Geometry check sheet. Reference: the model listing, model coordinates, mm. A direction names the side the tool comes from. Round coordinates to 2 decimals unless told otherwise and drop trailing zeros. Write each loop counter-clockwise with the first axis right and the second up, starting at its lowest first coordinate (ties: lowest second). Pieces come first, ordered by that corner, then holes. Notation, with made-up numbers: M 42.25,-24.5 L 48.25,-24.5 A31 cw 48.25,5.5 Z; hole C 9,66.5 d4. An arc over 180 degrees is marked long. Use a Markdown table: item, result.
```python
from build123d import *

# Parameters (mm, degrees)
BOSS_EXTRUDE1_DEPTH = 80
SKETCH2_R           = 25
CUT_EXTRUDE1_DEPTH  = 161
SKETCH3_R           = 15
CUT_EXTRUDE2_DEPTH  = 10


with BuildPart() as part:
    # Sketch1 → Boss-Extrude1 (new body)
    with BuildSketch(Plane.XY):
        Polygon((0, 0), (0, 480), (800, 480), (800, 400), (80, 400), (80, 0), align=None)
    extrude(amount=BOSS_EXTRUDE1_DEPTH)

    # Sketch2 → Cut-Extrude1 (cut)
    with BuildSketch(Plane.XY.offset(80)):
        with Locations((750, 440)):
            Circle(SKETCH2_R)
    extrude(amount=-CUT_EXTRUDE1_DEPTH, mode=Mode.SUBTRACT)

    # Sketch3 → Cut-Extrude2 (cut)
    with BuildSketch(Plane.XZ):
        with Locations(Location((40, 40, 0), (0, 0, 270))):
            Circle(SKETCH3_R)
    extrude(amount=-CUT_EXTRUDE2_DEPTH, mode=Mode.SUBTRACT)


solid = part.part
```
Item 1: Go/stop test with flat-tipped pins: pin 1 (8 mm diameter, centred on x = 398.5, z = 68, fed in from -Y); pin 2 (24 mm diameter, centred on y = 136, z = 44, fed in from +X); pin 3 (24 mm diameter, centred on x = 40, z = 40, fed in from -Y). Record where each tip stops, or that it passes through.
Outcome:
| item | result |
|---|---|
| pin 1 | stops at y = 400 |
| pin 2 | stops at x = 80 |
| pin 3 | stops at y = 10 |
Item 2: Cross-section at B-B, the plane z = 40. Record the cut outline in (x, y).
Outcome:
| item | result |
|---|---|
| outline | M 0,0 L 25,0 L 25,10 L 55,10 L 55,0 L 80,0 L 80,400 L 800,400 L 800,480 L 0,480 Z; hole C 750,440 d50 |
Item 3: Mould release check, pull along X, two halves, no side actions. Record for faces 4 (the face through (763.44, 461.08, 40.56)), 5 (the face through (800, 441, 39)), 6 (the face through (283, 401, 0)), 7 (the face through (0, 237, 39)): +X half, -X half, draft (parallel to the pull), parting line (faces both ways), or undercut.
Outcome:
| item | result |
|---|---|
| face 4 | undercut |
| face 5 | +X half |
| face 6 | draft |
| face 7 | -X half |
Item 4: Access from +Z, -Z, +X, -X, +Y, -Y to the whole of each face (thin tool, end or side, straight path). Record for faces 1 (the face through (50.138, 4.93, 51.056)), 2 (the face through (80, 203, 39)), 3 (the face through (394, 480, 39)).
Outcome:
| item | result |
|---|---|
| face 1 | -Y |
| face 2 | +Z, -Z, +X, -Y |
| face 3 | +Z, -Z, +X, -X, +Y |
Item 5: Material ranges on line 1 along X through (y, z) = (7.25, 40); line 2 along Y through (x, z) = (750, 47); line 3 along Y through (x, z) = (507, 53.5), recorded low to high. Write a range as from..to.
Outcome:
| item | result |
|---|---|
| line 1 | x = 0..25, 55..80 |
| line 2 | y = 400..415, 465..480 |
| line 3 | y = 400..480 |
Item 6: Cross-section at A-A, the plane y = 425. Record the cut outline in (x, z), and give its area (3 significant figures).
Outcome:
| item | result |
|---|---|
| outline | M 0,0 L 730,0 L 730,80 L 0,80 Z; M 770,0 L 800,0 L 800,80 L 770,80 Z |
| area | 60,800 mm2 |
Item 7: Cross-section at D-D, the plane y = 126. Record the cut outline in (x, z), and give its area (3 significant figures).
Outcome:
| item | result |
|---|---|
| outline | M 0,0 L 80,0 L 80,80 L 0,80 Z |
| area | 6,400 mm2 |
Item 8: Cross-section at C-C, the plane x = 750. Record the cut outline in (y, z), and give its area (3 significant figures).
Outcome:
| item | result |
|---|---|
| outline | M 400,0 L 415,0 L 415,80 L 400,80 Z; M 465,0 L 480,0 L 480,80 L 465,80 Z |
| area | 2,400 mm2 |
